from build123d import *

# Parameters (mm, degrees)
SKETCH1_R              = 50
BOSS_EXTRUDE1_DEPTH    = 3
SPLIT1_SURFACE_1_BACK  = 170.732
SPLIT1_SURFACE_1_DEPTH = 341.464
SPLIT1_SURFACE_2_BACK  = 170.732
SPLIT1_SURFACE_2_DEPTH = 341.464
BODY_DELETE1_DEPTH     = 3
FILLET1_R              = 3
BOSS_EXTRUDE4_DEPTH    = 3
SPLIT2_SURFACE_3_BACK  = 109.724
SPLIT2_SURFACE_3_DEPTH = 219.448
SPLIT2_SURFACE_4_BACK  = 109.724
SPLIT2_SURFACE_4_DEPTH = 219.448
FILLET2_R              = 3
SKETCH5_R              = 1
CUT_EXTRUDE1_DEPTH     = 3
SKETCH6_W              = 3
SKETCH6_H              = 10
BOSS_EXTRUDE5_DEPTH    = 3
BOSS_EXTRUDE6_DEPTH    = 3
SKETCH8_W              = 5
SKETCH8_H              = 3
BOSS_EXTRUDE7_DEPTH    = 3
SKETCH9_W              = 5
SKETCH9_H              = 4
CUT_EXTRUDE2_DEPTH     = 3


# Read off the part's stored shape, not the designer's step: Body-Delete1
with BuildPart() as part:
    # Sketch1 → Boss-Extrude1 (new body)
    with BuildSketch(Plane(origin=(0, 0, 0), x_dir=(1, 0, 0), z_dir=(0, 1, 0))):
        with BuildLine():
            ThreePointArc((10, 0), (-107.445626465, 17.320508076), (0, -33.166247904))
            Line((0, -33.166247904), (0, -60))
            Line((0, -60), (10, -60))
            Line((10, -60), (10, 0))
        make_face()
        with Locations(Location((-50, 0, 0), (0, 0, 270))):
            Circle(SKETCH1_R, mode=Mode.SUBTRACT)
    extrude(amount=BOSS_EXTRUDE1_DEPTH)


with BuildPart() as body_2:
    # Split1: the piece behind the surface
    add(part.part)
    # Split1 surface: a surface, the sketch's curves swept straight by 341.464 mm
    with BuildLine(Plane(origin=(0, 3, 0), x_dir=(1, 0, 0), z_dir=(0, 1, 0)).offset(-SPLIT1_SURFACE_1_BACK), mode=Mode.PRIVATE) as split1_surface_1_path:
        Line((0, -33.166247904), (0, 0))
        Line((0, 0), (-12, 0))
        Line((-12, 0), (-12, 32.496153619))
        Line((-12, 32.496153619), (-12, 67.159700612))
        Line((-12, 67.159700612), (-127.638562935, 67.159700612))
        Line((-127.638562935, 67.159700612), (-127.638562935, -72.196904976))
        Line((-127.638562935, -72.196904976), (0, -72.196904976))
        Line((0, -72.196904976), (0, -33.166247904))
    split1_surface_1 = Shell.extrude(split1_surface_1_path.wire(), (0 * SPLIT1_SURFACE_1_DEPTH, 1 * SPLIT1_SURFACE_1_DEPTH, 0 * SPLIT1_SURFACE_1_DEPTH))
    split(bisect_by=split1_surface_1, keep=Keep.BOTTOM)

    # Fillet1
    fillet1_edges = [body_2.edges().sort_by_distance(p)[0] for p in [
        (10, 1.5, 60),
    ]]
    fillet(fillet1_edges, radius=FILLET1_R)

    # Sketch3 → Boss-Extrude4 (add)
    with BuildSketch(Plane(origin=(0, 3, 0), x_dir=(1, 0, 0), z_dir=(0, 1, 0))):
        Polygon((0, -50), (-8, -50), (-8, -40), (0, -40), (3, -40), (3, -50), align=None)
        Polygon((-8, -20), (-8, -30), (0, -30), (3, -30), (3, -20), (0, -20), align=None)
    extrude(amount=-BOSS_EXTRUDE4_DEPTH)


with BuildPart() as part_1:
    add(part.part)

    # Split1: split by a surface, the side it looks to stays
    # Split1 surface: a surface, the sketch's curves swept straight by 341.464 mm
    with BuildLine(Plane(origin=(0, 3, 0), x_dir=(1, 0, 0), z_dir=(0, 1, 0)).offset(-SPLIT1_SURFACE_2_BACK), mode=Mode.PRIVATE) as split1_surface_2_path:
        Line((0, -33.166247904), (0, 0))
        Line((0, 0), (-12, 0))
        Line((-12, 0), (-12, 32.496153619))
        Line((-12, 32.496153619), (-12, 67.159700612))
        Line((-12, 67.159700612), (-127.638562935, 67.159700612))
        Line((-127.638562935, 67.159700612), (-127.638562935, -72.196904976))
        Line((-127.638562935, -72.196904976), (0, -72.196904976))
        Line((0, -72.196904976), (0, -33.166247904))
    split1_surface_2 = Shell.extrude(split1_surface_2_path.wire(), (0 * SPLIT1_SURFACE_2_DEPTH, 1 * SPLIT1_SURFACE_2_DEPTH, 0 * SPLIT1_SURFACE_2_DEPTH))
    split(bisect_by=split1_surface_2, keep=Keep.TOP)

    # Body-Delete1 outline → Body-Delete1 (cut)
    with BuildSketch(Plane(origin=(0, 0, 0), x_dir=(1, 0, 0), z_dir=(0, 1, 0))):
        with BuildLine():
            ThreePointArc((-12, 46.432747065), (-109.329587897, -8.94427191), (0, -33.166247904))
            Line((0, -33.166247904), (0, 0))
            ThreePointArc((0, 0), (-96.904157598, -17.320508075), (-12, 32.496153619))
            Line((-12, 32.496153619), (-12, 46.432747065))
        make_face()
    extrude(amount=BODY_DELETE1_DEPTH, mode=Mode.SUBTRACT)


with BuildPart() as body_2_2:
    # Split2: the piece behind the surface
    add(body_2.part)
    # Split2 surface: a surface, the sketch's curves swept straight by 219.448 mm
    with BuildLine(Plane(origin=(0, 3, 0), x_dir=(1, 0, 0), z_dir=(0, 1, 0)).offset(-SPLIT2_SURFACE_3_BACK), mode=Mode.PRIVATE) as split2_surface_3_path:
        Line((-12, 40.432747065), (-5.669502994, 40.432747065))
        Line((-5.669502994, 40.432747065), (-5.042290504, 40.432747065))
        Line((-5.042290504, 40.432747065), (-5.042290504, 47.453598883))
        Line((-5.042290504, 47.453598883), (-14.646815791, 47.453598883))
        Line((-14.646815791, 47.453598883), (-14.646815791, 40.432747065))
        Line((-14.646815791, 40.432747065), (-12, 40.432747065))
    split2_surface_3 = Shell.extrude(split2_surface_3_path.wire(), (0 * SPLIT2_SURFACE_3_DEPTH, 1 * SPLIT2_SURFACE_3_DEPTH, 0 * SPLIT2_SURFACE_3_DEPTH))
    split(bisect_by=split2_surface_3, keep=Keep.BOTTOM)

    # Fillet2
    fillet2_edges = [body_2_2.edges().sort_by_distance(p)[0] for p in [
        (-5.669502994, 1.5, -40.432747065),
    ]]
    fillet(fillet2_edges, radius=FILLET2_R)

    # Sketch5 → Cut-Extrude1 (cut)
    with BuildSketch(Plane(origin=(0, 3, 0), x_dir=(1, 0, 0), z_dir=(0, 1, 0))):
        with Locations(Location((-10, 38.432747065, 0), (0, 0, 270))):
            Circle(SKETCH5_R)
        with Locations(Location((-7, 35.432747065, 0), (0, 0, 270))):
            Circle(SKETCH5_R)
    extrude(amount=-CUT_EXTRUDE1_DEPTH, mode=Mode.SUBTRACT)

    # Sketch6 → Boss-Extrude5 (add)
    with BuildSketch(Plane(origin=(0, 3, 0), x_dir=(1, 0, 0), z_dir=(0, 1, 0))):
        with Locations((11.5, -35)):
            Rectangle(SKETCH6_W, SKETCH6_H)
        with Locations((11.5, -21)):
            Rectangle(SKETCH6_W, SKETCH6_H)
    extrude(amount=-BOSS_EXTRUDE5_DEPTH)

    # Sketch7 → Boss-Extrude6 (add)
    with BuildSketch(Plane(origin=(0, 3, 0), x_dir=(1, 0, 0), z_dir=(0, 1, 0))):
        Polygon((-5.328723834, -40), (-5.328723834, -37), (0, -37), (1.654581998, -37), (1.654581998, -41.537905148), (-0.328723834, -41.537905148), (-5.328723834, -41.537905148), align=None)
        Polygon((-5.328723834, -50), (-5.328723834, -53), (0, -53), (1.654581998, -53), (1.654581998, -47.713051581), (-5.328723834, -47.713051581), align=None)
    extrude(amount=-BOSS_EXTRUDE6_DEPTH)

    # Sketch8 → Boss-Extrude7 (add)
    with BuildSketch(Plane(origin=(0, 3, 0), x_dir=(1, 0, 0), z_dir=(0, 1, 0))):
        with Locations((-2.5, -18.5)):
            Rectangle(SKETCH8_W, SKETCH8_H)
        with Locations((-2.5, -31.5)):
            Rectangle(SKETCH8_W, SKETCH8_H)
    extrude(amount=-BOSS_EXTRUDE7_DEPTH)

    # Sketch9 → Cut-Extrude2 (cut)
    with BuildSketch(Plane(origin=(0, 3, 0), x_dir=(1, 0, 0), z_dir=(0, 1, 0))):
        with Locations((-2.5, -25)):
            Rectangle(SKETCH9_W, SKETCH9_H)
        with Locations((-2.5, -45)):
            Rectangle(SKETCH9_W, SKETCH9_H)
    extrude(amount=-CUT_EXTRUDE2_DEPTH, mode=Mode.SUBTRACT)


with BuildPart() as body_2_1:
    add(body_2.part)

    # Split2: split by a surface, the side it looks to stays
    # Split2 surface: a surface, the sketch's curves swept straight by 219.448 mm
    with BuildLine(Plane(origin=(0, 3, 0), x_dir=(1, 0, 0), z_dir=(0, 1, 0)).offset(-SPLIT2_SURFACE_4_BACK), mode=Mode.PRIVATE) as split2_surface_4_path:
        Line((-12, 40.432747065), (-5.669502994, 40.432747065))
        Line((-5.669502994, 40.432747065), (-5.042290504, 40.432747065))
        Line((-5.042290504, 40.432747065), (-5.042290504, 47.453598883))
        Line((-5.042290504, 47.453598883), (-14.646815791, 47.453598883))
        Line((-14.646815791, 47.453598883), (-14.646815791, 40.432747065))
        Line((-14.646815791, 40.432747065), (-12, 40.432747065))
    split2_surface_4 = Shell.extrude(split2_surface_4_path.wire(), (0 * SPLIT2_SURFACE_4_DEPTH, 1 * SPLIT2_SURFACE_4_DEPTH, 0 * SPLIT2_SURFACE_4_DEPTH))
    split(bisect_by=split2_surface_4, keep=Keep.TOP)


solid = body_2_2.part
Verification items for the finished model (mm, model axes). A direction names the side the tool comes from. Give positions to 0.01 mm unless a question says otherwise; leave off trailing zeros. Write each loop counter-clockwise with the first axis right and the second up, starting at its lowest first coordinate (ties: lowest second). Pieces come first, ordered by that corner, then holes. Notation, with made-up numbers: (-25, -30.75) - (-7, -30.75) arc R15 ccw to (-7, -20.75) - close; hole circle Ø4 at (85.25, -25.5). An arc over 180 degrees is marked (long way). Answer as CSV lines item,"result". Start each with the question number.
1. Sectioned sample at B-B (y = 2.4). Count the separate pieces of the cut face and the enclosed holes in it, then the cut area to 3 significant figures.
2. Sectioned sample at D-D (z = 21.5). Record the boundary of the cut face in (x, y), then the cut area to 3 significant figures.
3. Thickness scan on line 1 (Z direction, x = 11, y = 0.9); line 2 (X direction, y = 1.2, z = 32); line 3 (X direction, y = 1.15, z = 15). Record the ranges inside material, lowest first.
4. Draft check along X on faces 1 (the face through (11, 2, 26)), 2 (the face through (6.296, 1.479, -20.755)), 3 (the face through (0, 2, 45)), 4 (the face through (-5, 2, 45)). Enter one of: pulls with the +X half, pulls with the -X half, needs draft (parallel to the pull), parting line crosses it, or undercut.
5. Sectioned sample at C-C (x = -3.5). Record the boundary of the cut face in (y, z), then the cut area to 3 significant figures.
6. Sectioned sample at A-A (x = -10). Record the boundary of the cut face in (y, z), then the cut area to 3 significant figures.
7. Set-up check for faces 5 (the face through (-8, 2, 45)), 6 (the face through (11, 2, 40)), 7 (the face through (-3, 2, 37)): record each of +Z, -Z, +X, -X, +Y, -Y from which the full face is reachable in a straight line by a thin tool's end or side.
8. Depth check by flat-ended pin: pin 1 (1 mm diameter, centred on x = -3, y = 2.5, fed in from -Z); pin 2 (1.5 mm diameter, centred on y = 1.5, z = 18, fed in from -X); pin 3 (1.5 mm diameter, centred on x = -7, y = 2, fed in from +Z); pin 4 (2 mm diameter, centred on x = -6, z = 24, fed in from -Y). Enter the tip coordinate at first touch or a pass-through.
Derived:
1,separate pieces,"1"
1,enclosed holes,"4"
1,area,"1,260 mm²"
2,outline,"(-8, 0) - (13, 0) - (13, 3) - (-8, 3) - close"
2,area,"63.0 mm²"
3,line 1,"16 to 26, 30 to 40"
3,line 2,"-5 to 13"
3,line 3,"0 to 10"
4,face 1,"needs draft"
4,face 2,"pulls with the +X half"
4,face 3,"undercut"
4,face 4,"undercut"
5,outline,"(0, -37.92) - (3, -37.92) - (3, -18.38) - (0, -18.38) - close; (0, 17) - (3, 17) - (3, 23) - (0, 23) - close; (0, 27) - (3, 27) - (3, 33) - (0, 33) - close; (0, 37) - (3, 37) - (3, 43) - (0, 43) - close; (0, 47) - (3, 47) - (3, 53) - (0, 53) - close"
5,area,"131 mm²"
6,outline,"(0, -40.43) - (3, -40.43) - (3, -39.43) - (0, -39.43) - close; (0, -37.43) - (3, -37.43) - (3, -30) - (0, -30) - close"
6,area,"25.3 mm²"
7,face 5,"+Z, -X, +Y, -Y"
7,face 6,"+Z, +X, +Y, -Y"
7,face 7,"-X, +Y, -Y"
8,pin 1,"z = -37.92"
8,pin 2,"x = -5"
8,pin 3,"z = 50"
8,pin 4,"y = 0"
